The model under review builds one solid part; all positions refer to its coordinate system, in mm. Give positions to 0.01 mm unless a question says otherwise; leave off trailing zeros. Order: outer loops, then holes, each group sorted by start corner. A loop starts at its lowest first (then second) coordinate and runs counter-clockwise, first axis right, second up.
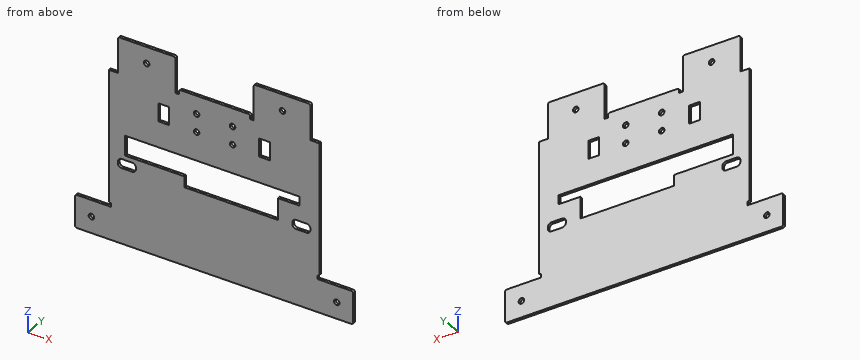
Autodesk Inventor part; units mm, degrees
ref_plane "YZ Plane" through (0, 0, 0) normal (1, 0, 0) x (0, 1, 0)
ref_plane "XZ Plane" through (0, 0, 0) normal (0, 1, 0) x (-1, 0, 0)
ref_plane "XY Plane" through (0, 0, 0) normal (0, 0, 1) x (1, 0, 0)
sketch "Sketch1" plane through (0, 0, 0) normal (0, 1, 0) x (-1, 0, 0)
  line L0 (112, 55.3296) -> (80, 55.3296)
  line L1 (117.1396, -39.0893) -> (117.1396, -20.8993)
  line L2 (117, -0.4496) -> (0, -0.4496)
  line L3 (36.5, 55.3296) -> (5, 55.3296)
  line L4 (-0.1396, -20.8993) -> (-0.1396, -39.0893)
  circle A0 centre (48.25, 46.69) radius 1.55
  circle A1 centre (48.25, 36.69) radius 1.55
  circle A2 centre (68.25, 46.69) radius 1.55
  circle A3 centre (68.25, 36.69) radius 1.55
  line L5 (83.46, 35.26) -> (83.46, 45.26)
  line L6 (89.46, 35.26) -> (83.46, 35.26)
  line L7 (89.46, 45.26) -> (89.46, 35.26)
  line L8 (83.46, 45.26) -> (89.46, 45.26)
  line L9 (33.54, 45.26) -> (33.54, 35.26)
  line L10 (27.54, 45.26) -> (33.54, 45.26)
  line L11 (27.54, 35.26) -> (27.54, 45.26)
  line L12 (33.54, 35.26) -> (27.54, 35.26)
  line L13 (108, 21) -> (108, 10)
  line L14 (11, 21) -> (108, 21)
  line L15 (11, 16) -> (11, 21)
  line L16 (23, 16) -> (11, 16)
  line L17 (23, 4) -> (23, 16)
  line L18 (75, 4) -> (23, 4)
  line L19 (75, 10) -> (75, 4)
  line L20 (108, 10) -> (75, 10)
  arc A4 (112, 5.5) -> (110, 7.5) centre (110, 5.5) ccw
  line L21 (104, 7.5) -> (110, 7.5)
  arc A5 (110, 2.5) -> (112, 4.5) centre (110, 4.5) ccw
  line L22 (110, 2.5) -> (104, 2.5)
  arc A6 (102, 4.5) -> (104, 2.5) centre (104, 4.5) ccw
  line L23 (102, 4.5) -> (102, 5.5)
  arc A7 (104, 7.5) -> (102, 5.5) centre (104, 5.5) ccw
  arc A8 (15, 5.5) -> (13, 7.5) centre (13, 5.5) ccw
  line L24 (7, 7.5) -> (13, 7.5)
  arc A9 (13, 2.5) -> (15, 4.5) centre (13, 4.5) ccw
  line L25 (13, 2.5) -> (7, 2.5)
  arc A10 (5, 4.5) -> (7, 2.5) centre (7, 4.5) ccw
  line L26 (5, 4.5) -> (5, 5.5)
  arc A11 (7, 7.5) -> (5, 5.5) centre (7, 5.5) ccw
  line L27 (112, 5.5) -> (112, 4.5)
  line L28 (15, 5.5) -> (15, 4.5)
  circle A12 centre (20.5, 64.8743) radius 1.55
  circle A13 centre (96, 64.8743) radius 1.55
  circle A14 centre (-9.6843, -29.9943) radius 1.55
  circle A15 centre (126.6843, -29.9943) radius 1.55
  arc A16 (0, -17.8993) -> (1, -18.8993) centre (1, -17.8993) ccw
  arc A17 (116, -18.8993) -> (117, -17.8993) centre (116, -17.8993) ccw
  line L29 (115.94, -18.8993) -> (116, -18.8993)
  arc A18 (135.7793, -21.8993) -> (134.7793, -20.8993) centre (134.7793, -21.8993) ccw
  arc A19 (134.7793, -39.0893) -> (135.7793, -38.0893) centre (134.7793, -38.0893) ccw
  line L30 (134.7793, -39.0893) -> (-17.7793, -39.0893)
  arc A20 (-18.7793, -38.0893) -> (-17.7793, -39.0893) centre (-17.7793, -38.0893) ccw
  arc A21 (-17.7793, -20.8993) -> (-18.7793, -21.8993) centre (-17.7793, -21.8993) ccw
  line L31 (-17.7793, -20.8993) -> (1.06, -20.8993)
  arc A22 (39.5, 56.69) -> (38.5, 55.69) centre (39.5, 55.69) ccw
  line L32 (39.5, 56.69) -> (77, 56.69)
  arc A23 (78, 55.69) -> (77, 56.69) centre (77, 55.69) ccw
  arc A24 (81, 73.9693) -> (80, 72.9693) centre (81, 72.9693) ccw
  arc A25 (112, 72.9693) -> (111, 73.9693) centre (111, 72.9693) ccw
  arc A26 (6, 73.9693) -> (5, 72.9693) centre (6, 72.9693) ccw
  arc A27 (36.5, 72.9693) -> (35.5, 73.9693) centre (35.5, 72.9693) ccw
  line L33 (36.5, 72.9693) -> (36.5, 54.13)
  line L34 (6, 73.9693) -> (35.5, 73.9693)
  line L35 (38.5, 55.69) -> (38.5, 54.13)
  line L36 (38.5, 54.13) -> (36.5, 54.13)
  line L37 (5, 54.13) -> (5, 72.9693)
  line L38 (5, 54.13) -> (0, 54.13)
  line L39 (0, -17.8993) -> (0, 54.13)
  line L40 (81, 73.9693) -> (111, 73.9693)
  line L41 (112, 54.13) -> (112, 72.9693)
  line L42 (117, 54.13) -> (112, 54.13)
  line L43 (78, 54.13) -> (78, 55.69)
  line L44 (80, 72.9693) -> (80, 54.13)
  line L45 (80, 54.13) -> (78, 54.13)
  line L46 (117, 54.13) -> (117, -17.8993)
  line L47 (-18.7793, -38.0893) -> (-18.7793, -21.8993)
  line L48 (135.7793, -21.8993) -> (135.7793, -38.0893)
  line L49 (115.94, -20.8993) -> (134.7793, -20.8993)
  line L50 (115.94, -20.8993) -> (115.94, -18.8993)
  line L51 (1, -18.8993) -> (1.06, -18.8993)
  line L52 (1.06, -18.8993) -> (1.06, -20.8993)
  line L53 (-0.5893, -39.0893) -> (-0.5893, -20.8993)
  line L54 (117.5893, -20.8993) -> (117.5893, -39.0893)
  line L55 (0.31, -20.8993) -> (0.31, -39.0893)
  line L56 (116.69, -39.0893) -> (116.69, -20.8993)
  line L57 (5, 55.7793) -> (36.5, 55.7793)
  line L58 (117, -0.8993) -> (0, -0.8993)
  line L59 (80, 55.7793) -> (112, 55.7793)
  line L60 (36.5, 54.88) -> (5, 54.88)
  line L61 (0, 0) -> (117, 0)
  line L62 (112, 54.88) -> (80, 54.88)
extrude "Extrusion1" add sketch "Sketch1" against normal blind 1.5
properties part number "body_top_frame"
Item 1: Take a section at B-B (x = -48.25). Give the boundary of the cut face in (y, z).
Values found:
outline: (-1.5, -39.09) - (0, -39.09) - (0, 4) - (-1.5, 4) - close; (-1.5, 21) - (0, 21) - (0, 35.14) - (-1.5, 35.14) - close; (-1.5, 38.24) - (0, 38.24) - (0, 45.14) - (-1.5, 45.14) - close; (-1.5, 48.24) - (0, 48.24) - (0, 56.69) - (-1.5, 56.69) - close
Item 2: Take a section at D-D (x = -20.5). Give the boundary of the cut face in (y, z), and give its area (3 significant figures).
Values found:
outline: (-1.5, -39.09) - (0, -39.09) - (0, 16) - (-1.5, 16) - close; (-1.5, 21) - (0, 21) - (0, 63.32) - (-1.5, 63.32) - close; (-1.5, 66.42) - (0, 66.42) - (0, 73.97) - (-1.5, 73.97) - close
area: 157 mm2
Item 3: For line 1 (Z direction, x = -68, y = -0.15); line 2 (Z direction, x = -20.5, y = -1.15); line 3 (Z direction, x = -68.25, y = -0.8), list the stretches that pass through material, from the lowest coordinate up.
Values found:
line 1: z = -39.09 to 4, 21 to 35.16, 38.22 to 45.16, 48.22 to 56.69
line 2: z = -39.09 to 16, 21 to 63.32, 66.42 to 73.97
line 3: z = -39.09 to 4, 21 to 35.14, 38.24 to 45.14, 48.24 to 56.69
Item 4: Take a section at A-A (x = -96). Give the boundary of the cut face in (y, z), and give its area (3 significant figures).
Values found:
outline: (-1.5, -39.09) - (0, -39.09) - (0, 10) - (-1.5, 10) - close; (-1.5, 21) - (0, 21) - (0, 63.32) - (-1.5, 63.32) - close; (-1.5, 66.42) - (0, 66.42) - (0, 73.97) - (-1.5, 73.97) - close
area: 148 mm2
Item 5: Clearance check with a flat-ended pin moving along its axis: pin 1 Ø0.8 at (y, z) = (-1, 5) entering from +X. State where the tip first meets the part, or that it passes through.
Values found:
pin 1: stops at x = 0
Item 6: Take a section at C-C (z = 23). Give the boundary of the cut face in (x, y), and give its area (4 significant figures).
Values found:
outline: (-117, -1.5) - (0, -1.5) - (0, 0) - (-117, 0) - close
area: 175.5 mm2
